from build123d import *

# Parameters (mm, degrees)
SKETCH_1_R          = 17.8
EXTRUDE_1_DEPTH     = 2
SKETCH_2_R          = 7.85
EXTRUDE_2_DEPTH     = 0.8
DRAFT_1_ANGLE       = 1
SKETCH_38_R         = 4.8
EXTRUDE_3_DEPTH     = 1.9
SKETCH_39_R         = 5.25
EXTRUDE_4_DEPTH     = 0.4
SKETCH_40_R         = 1.5
CUT_EXTRUDE_1_DEPTH = 10.4
SKETCH_42_R         = 1.5
CUT_EXTRUDE_3_DEPTH = 10


with BuildPart() as part:
    # ｽｹｯﾁ1 → ﾎﾞｽ - 押し出し1 (new body)
    with BuildSketch(Plane.XY):
        Circle(SKETCH_1_R)
    extrude(amount=EXTRUDE_1_DEPTH)

    # ｽｹｯﾁ2 → ﾎﾞｽ - 押し出し2 (add)
    with BuildSketch(Plane(origin=(0, 0, 0), x_dir=(-1, 0, 0), z_dir=(0, 0, -1))):
        Circle(SKETCH_2_R)
    extrude(amount=EXTRUDE_2_DEPTH)

    # 抜き勾配1
    draft_1_faces = [part.faces().sort_by_distance(p)[0] for p in [
        (7.85, 0, -0.4),
    ]]
    draft(draft_1_faces, Plane(origin=(0, 0, -0.8), x_dir=(-1, 0, 0), z_dir=(0, 0, -1)), DRAFT_1_ANGLE)

    # ｽｹｯﾁ38 → ﾎﾞｽ - 押し出し3 (add)
    with BuildSketch(Plane(origin=(0, 0, -0.8), x_dir=(-1, 0, 0), z_dir=(0, 0, -1))):
        Circle(SKETCH_38_R)
    extrude(amount=EXTRUDE_3_DEPTH)

    # ｽｹｯﾁ39 → ﾎﾞｽ - 押し出し4 (add)
    with BuildSketch(Plane.XY.offset(2)):
        Circle(SKETCH_39_R)
    extrude(amount=EXTRUDE_4_DEPTH)

    # ｽｹｯﾁ40 → ｶｯﾄ - 押し出し1 (cut)
    with BuildSketch(Plane.XY.offset(2.4)):
        Circle(SKETCH_40_R)
    extrude(amount=-CUT_EXTRUDE_1_DEPTH, mode=Mode.SUBTRACT)

    # ｽｹｯﾁ42 → ｶｯﾄ - 押し出し3 (cut)
    with BuildSketch(Plane.XY.offset(2)):
        with Locations((0, 11)):
            Circle(SKETCH_42_R)
        with Locations((0, -11)):
            Circle(SKETCH_42_R)
    extrude(amount=-CUT_EXTRUDE_3_DEPTH, mode=Mode.SUBTRACT)


solid = part.part
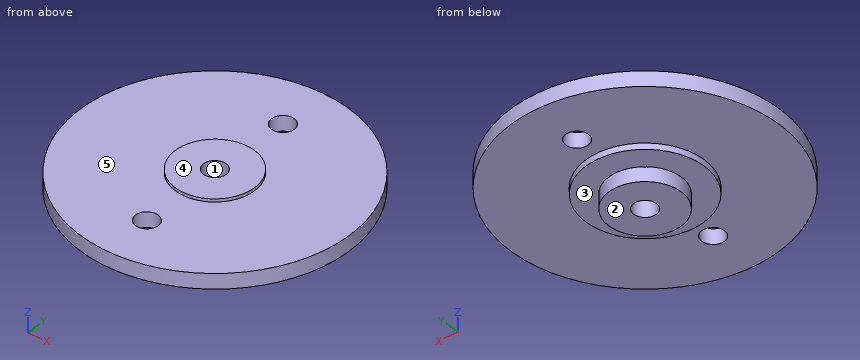
Source: CAD feature listing. Evaluate the final solid. Frame: model axes, mm. Face numbers are marked on the shaded views. A direction names the side the tool comes from. Coordinates: 2 decimals unless noted, no trailing zeros. Loops run counter-clockwise (first coordinate to the right, second up) from the corner with the lowest first, then second, coordinate; pieces in that order, holes last. Notation, with made-up numbers: (85, 87.5) - (104, 87.5) arc R26 cw to (104, 103.5) - close; hole circle Ø3 at (29, -6). An arc over 180 degrees is marked (long way). One line per item, written item: value. Start each with the question number.
1. Mould query, pull axis Y, two halves, no side actions, for the marked faces 1 and 2. Classes: pulls with the +Y half, pulls with the -Y half, needs draft (parallel to the pull), parting line crosses it, or undercut.
2. Section B-B (z = 1.3). Return the cut outline in (x, y), and give its area (3 significant figures).
3. Set-up query: the marked faces 3, 4 and 5. Return all of +Z, -Z, +X, -X, +Y, -Y with unobstructed straight access to the full face (end or side cutting, diameter ignored); none if empty.
4. Contact query for flat-ended pins moving along their axis: P1, Ø1, axis at x = 14, y = 6, coming from the -Z side; P2, Ø2, axis at x = -8.5, z = 0, coming from the +Y side; P3, Ø3, axis at x = 4, y = 8.5, coming from the +Z side; P4, Ø4, axis at x = 0, y = 0, coming from the -Z side. Output: stop coordinate, or through.
5. Section D-D (x = -13.5). Return the cut outline in (y, z), and give its area (3 significant figures).
6. Section C-C (x = 0). State how many separate pieces and enclosed holes the cut face has, and give its area (3 significant figures).
7. Ray query, L1, parallel to Y at x = 0, z = 0.85; L2, parallel to Y at x = 0, z = -1.25; L3, parallel to Z at x = 11, y = 12.5. Return the intervals inside material, ascending.
8. Section A-A (y = -11). Return the cut outline in (x, z).
Verdict:
1. face 1: undercut
1. face 2: needs draft
2. outline: circle Ø35.6 at (0, 0); hole circle Ø3 at (0, -11); hole circle Ø3 at (0, 0); hole circle Ø3 at (0, 11)
2. area: 974 mm2
3. face 3: -Z
3. face 4: +Z, +X, -X, +Y, -Y
3. face 5: +Z
4. P1: stops at z = 0
4. P2: stops at y = 16.14
4. P3: stops at z = 2
4. P4: stops at z = -2.7
5. outline: (-11.6, 0) - (11.6, 0) - (11.6, 2) - (-11.6, 2) - close
5. area: 46.4 mm2
6. separate pieces: 4
6. enclosed holes: 0
6. area: 78.9 mm2
7. L1: y = -17.8 to -12.5, -9.5 to -1.5, 1.5 to 9.5, 12.5 to 17.8
7. L2: y = -4.8 to -1.5, 1.5 to 4.8
7. L3: z = 0 to 2
8. outline: (-13.99, 0) - (-1.5, 0) - (-1.5, 2) - (-13.99, 2) - close; (1.5, 0) - (13.99, 0) - (13.99, 2) - (1.5, 2) - close
